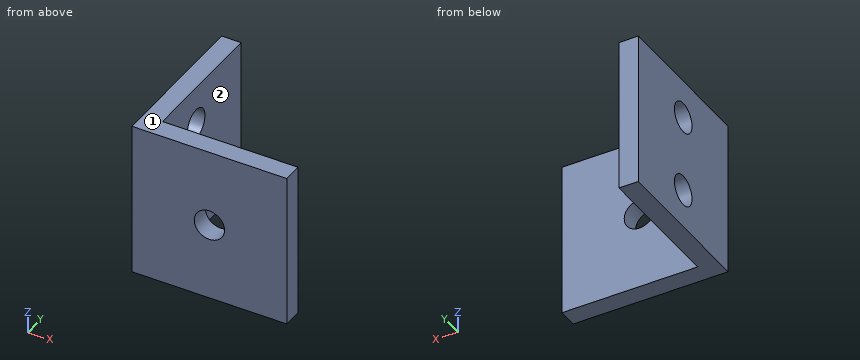
```python
from build123d import *

# Parameters (mm, degrees)
BOSS_EXTRUDE1_DEPTH     = 12.7
CUT_EXTRUDE1_DEPTH      = 37.061067996
CUT_EXTRUDE1_DEPTH_BACK = 37.061067996
SKETCH3_R               = 2.4892
CUT_EXTRUDE2_DEPTH      = 37.061067996
CUT_EXTRUDE2_DEPTH_BACK = 37.061067996
SKETCH4_R               = 2.4892


with BuildPart() as part:
    # Sketch1 → Boss-Extrude1 (new, symmetric)
    with BuildSketch(Plane.XY):
        Polygon((0, 0), (0, 25.4), (3.175, 25.4), (3.175, 3.175), (25.4, 3.175), (25.4, 0), align=None)
    extrude(amount=BOSS_EXTRUDE1_DEPTH, both=True)

    # Sketch3 → Cut-Extrude1 (cut, two sides: drawn at the far end of the back side and taken through both)
    with BuildSketch(Plane(origin=(0, 3.175, 0), x_dir=(1, 0, 0), z_dir=(0, 1, 0)).offset(-CUT_EXTRUDE1_DEPTH_BACK)):
        with Locations(Location((12.7, 0, 0), (0, 0, 270))):
            Circle(SKETCH3_R)
    extrude(amount=CUT_EXTRUDE1_DEPTH + CUT_EXTRUDE1_DEPTH_BACK, mode=Mode.SUBTRACT)

    # Sketch4 → Cut-Extrude2 (cut, two sides: drawn at the far end of the back side and taken through both)
    with BuildSketch(Plane(origin=(3.175, 0, 0), x_dir=(0, 0, -1), z_dir=(1, 0, 0)).offset(-CUT_EXTRUDE2_DEPTH_BACK)):
        with Locations(Location((-6.35, 12.7, 0), (0, 0, 90))):
            Circle(SKETCH4_R)
        with Locations(Location((6.35, 12.7, 0), (0, 0, 90))):
            Circle(SKETCH4_R)
    extrude(amount=CUT_EXTRUDE2_DEPTH + CUT_EXTRUDE2_DEPTH_BACK, mode=Mode.SUBTRACT)


solid = part.part
```
CAD build for the part. Positions are in the model's coordinates, mm. Face numbers are marked on the shaded views. A direction names the side the tool comes from. Coordinates: 2 decimals unless noted, no trailing zeros. Loops run counter-clockwise (first coordinate to the right, second up) from the corner with the lowest first, then second, coordinate; pieces in that order, holes last. Notation, with made-up numbers: (4, -11.75) - (14, -11.75) arc R8 ccw to (14, -5.75) - close; hole circle Ø8 at (60.25, 41.5). An arc over 180 degrees is marked (long way). Use CSV: the item, a comma, the result in double quotes. Start each with the question number.
Q1. Cut at A-A, the plane x = 12.7. List the corners of the cut face in (y, z) (3 decimals).
Q2. Cut at B-B, the plane z = -6.35. List the corners of the cut face in (x, y) (3 decimals), then the cut area to 3 significant figures.
Q3. Probe probe 1 along Z at (x, y) = (0.7, 12.7); probe 2 along X at (y, z) = (0.85, 0). List the from-to ranges inside material, lowest first. Write a range as from..to.
Q4. Cut at D-D, the plane z = 11.25. List the corners of the cut face in (x, y) (3 decimals).
Q5. Cut at C-C, the plane y = 20. List the corners of the cut face in (x, z) (3 decimals).
Q6. 3-axis set-ups, long thin cutter, end or side, ignore diameter. For the marked faces 1 and 2: which of +Z, -Z, +X, -X, +Y, -Y reach the whole face in a straight line?
Q7. Drop flat-ended pins along their axis: P1, Ø3, axis at y = 14.5, z = -5.5, coming from the +X side (3 decimals); P2, Ø11, axis at x = 16.5, z = 2.5, coming from the +Y side (3 decimals). Give the stop position or say it passes through.
Here are the results:
1,outline,"(0, -12.7) - (3.175, -12.7) - (3.175, -2.489) - (0, -2.489) - close; (0, 2.489) - (3.175, 2.489) - (3.175, 12.7) - (0, 12.7) - close"
2,outline,"(0, 0) - (25.4, 0) - (25.4, 3.175) - (3.175, 3.175) - (3.175, 10.211) - (0, 10.211) - close; (0, 15.189) - (3.175, 15.189) - (3.175, 25.4) - (0, 25.4) - close"
2,area,"135 mm2"
3,probe 1,"-12.7..-8.84, -3.86..3.86, 8.84..12.7"
3,probe 2,"0..10.21, 15.19..25.4"
4,outline,"(0, 0) - (25.4, 0) - (25.4, 3.175) - (3.175, 3.175) - (3.175, 25.4) - (0, 25.4) - close"
5,outline,"(0, -12.7) - (3.175, -12.7) - (3.175, 12.7) - (0, 12.7) - close"
6,face 1,"+Z, +X, -X, +Y, -Y"
6,face 2,"+Z, -Z, +X, +Y"
7,P1,"x = 3.175"
7,P2,"y = 3.175"
